CAD build for the part. Positions are in the model's coordinates, mm. Round coordinates to 2 decimals unless told otherwise and drop trailing zeros. Write each loop counter-clockwise with the first axis right and the second up, starting at its lowest first coordinate (ties: lowest second). Pieces come first, ordered by that corner, then holes. Notation, with made-up numbers: (11, 12) - (33, 12) arc R23 cw to (33, 29) - close; hole circle Ø11 at (19, 81). An arc over 180 degrees is marked (long way). Use one line per item in the form item = value. Start each with the question number.
Item 1: Band-saw the part on A-A, the plane z = 0. List the corners of the cut face in (x, y), and give its area (3 significant figures).
Item 2: Pin check, flat tips, straight feed: pin 1 (1.5 mm diameter, centred on x = 27, z = 27.5, fed in from -Y); pin 2 (1.4 mm diameter, centred on y = 412, z = -39, fed in from +X); pin 3 (5 mm diameter, centred on y = 623, z = 14.5, fed in from +X); pin 4 (5 mm diameter, centred on x = 23.5, y = 538.5, fed in from -Z). Stop position of each tip, or through.
Item 3: Band-saw the part on D-D, the plane z = -29. List the corners of the cut face in (x, y), and give its area (3 significant figures).
Item 4: Drill centre lines: L1, parallel to X at y = 252, z = 0; L2, parallel to X at y = 80, z = -14.5. Where is each one in solid material? Low to high.
Item 5: Band-saw the part on C-C, the plane y = 95.5. List the corners of the cut face in (x, z).
Item 6: Band-saw the part on B-B, the plane x = 14.5. List the corners of the cut face in (y, z), and give its area (3 significant figures).
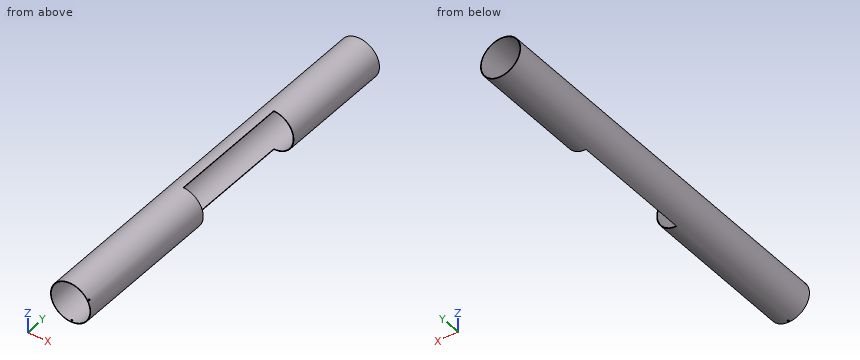
from build123d import *

# Parameters (mm, degrees)
SKETCH1_R           = 39.37
SKETCH1_R_2         = 38.1
BOSS_EXTRUDE1_DEPTH = 762
SKETCH2_R           = 1.692869147
CUT_EXTRUDE1_DEPTH  = 61.4
CIRPATTERN3_COUNT   = 3
SKETCH4_W           = 96.846889453
SKETCH4_H           = 239.152522935
CUT_EXTRUDE3_DEPTH  = 200


with BuildPart() as part:
    # Sketch1 → Boss-Extrude1 (new body)
    with BuildSketch(Plane(origin=(0, 0, 0), x_dir=(1, 0, 0), z_dir=(0, 1, 0))):
        with Locations(Location((0, 0, 0), (0, 0, 270))):
            Circle(SKETCH1_R)
        with Locations(Location((0, 0, 0), (0, 0, 270))):
            Circle(SKETCH1_R_2, mode=Mode.SUBTRACT)
    extrude(amount=BOSS_EXTRUDE1_DEPTH)

    # Sketch2 → Cut-Extrude1 (cut)
    with BuildSketch(Plane.XY):
        with Locations(Location((0, 3.287142885, 0), (0, 0, 90))):
            Circle(SKETCH2_R)
    cut_extrude1 = extrude(amount=-CUT_EXTRUDE1_DEPTH, mode=Mode.SUBTRACT)

    # CirPattern3: Cut-Extrude1 ×3 about axis
    cirpattern3_axis = Axis((0, 0, 0), (0, -1, 0))
    for i in range(1, CIRPATTERN3_COUNT):
        add(cut_extrude1.rotate(cirpattern3_axis, i * 360 / CIRPATTERN3_COUNT), mode=Mode.SUBTRACT)

    # Sketch4 → Cut-Extrude3 (cut)
    with BuildSketch(Plane(origin=(0, 0, 0), x_dir=(0, 0, -1), z_dir=(1, 0, 0))):
        with Locations((-1.346410096, 416.735952277)):
            Rectangle(SKETCH4_W, SKETCH4_H)
    extrude(amount=CUT_EXTRUDE3_DEPTH, mode=Mode.SUBTRACT)


solid = part.part
Determined:
q1.outline = (-39.37, 0) - (-38.1, 0) - (-38.1, 762) - (-39.37, 762) - close; (38.1, 0) - (39.37, 0) - (39.37, 297.16) - (38.1, 297.16) - close; (38.1, 536.31) - (39.37, 536.31) - (39.37, 762) - (38.1, 762) - close
q1.area = 1,630 mm²
q2.pin_1 = 0
q2.pin_2 = 0
q2.pin_3 = 37.5
q2.pin_4 = -33.3
q3.outline = (-26.63, 0) - (-24.71, 0) - (-24.71, 762) - (-26.63, 762) - close; (24.71, 0) - (26.63, 0) - (26.63, 297.16) - (24.71, 297.16) - close; (24.71, 536.31) - (26.63, 536.31) - (26.63, 762) - (24.71, 762) - close
q3.area = 2,460 mm²
q4.L1 = -39.37 to -38.1, 38.1 to 39.37
q4.L2 = -36.6 to -35.23, 35.23 to 36.6
q5.outline = circle Ø78.74 at (0, 0); hole circle Ø76.2 at (0, 0)
q6.outline = (0, -36.6) - (297.16, -36.6) - (297.16, -35.23) - (0, -35.23) - close; (0, 35.23) - (297.16, 35.23) - (297.16, 36.6) - (0, 36.6) - close; (536.31, -36.6) - (762, -36.6) - (762, -35.23) - (536.31, -35.23) - close; (536.31, 35.23) - (762, 35.23) - (762, 36.6) - (536.31, 36.6) - close
q6.area = 1,430 mm²
